Geometry check sheet. Reference: the model listing, model coordinates, mm. Round coordinates to 2 decimals unless told otherwise and drop trailing zeros. Loops run counter-clockwise (first coordinate to the right, second up) from the corner with the lowest first, then second, coordinate; pieces in that order, holes last. Notation, with made-up numbers: (44, -16) -> (64, -16) arc R15 ccw to (64, -8) -> close; hole circle Ø3 at (-32, 88.25). An arc over 180 degrees is marked (long way). Use one line per item in the form item = value.
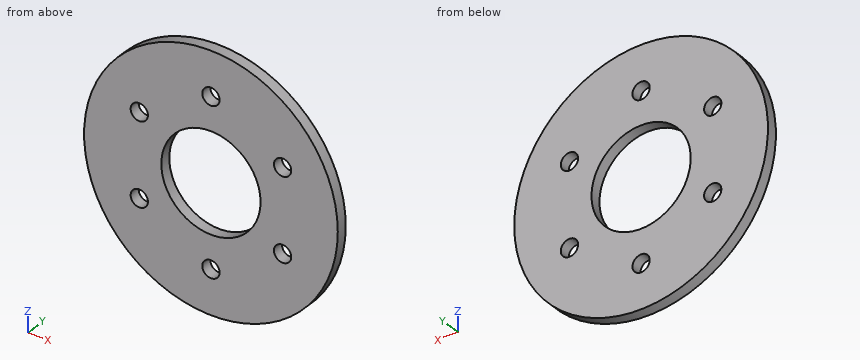
from build123d import *

# Parameters (mm, degrees)
F0_R            = 36.5125
F0_R_2          = 14.2875
F1_DEPTH        = 3.175
F2_R            = 2.4892
F3_DEPTH        = 3.176
F3_COPIES_COUNT = 6


# Not quite as in the source:
# - a pattern or mirror of a feature is missing from the dataset's text; its kind, count and spacing are read off the source's solid


with BuildPart() as f1:
    # F0 (on Front) → F1 (new body)
    with BuildSketch(Plane.XZ):
        Circle(F0_R)
        Circle(F0_R_2, mode=Mode.SUBTRACT)
    extrude(amount=F1_DEPTH)

    # F2 (on face) → F3 (cut, through all)
    with BuildSketch(Plane.XZ.offset(3.175)):
        with Locations((0, 23.8125)):
            Circle(F2_R)
    f3 = extrude(amount=-F3_DEPTH, mode=Mode.SUBTRACT)

    # F3_copies: F3 ×6 about axis
    f3_copies_axis = Axis((0, 0, 0), (0, 1, 0))
    for i in range(1, F3_COPIES_COUNT):
        add(f3.rotate(f3_copies_axis, i * 360 / F3_COPIES_COUNT), mode=Mode.SUBTRACT)


solid = f1.part
1. Section check A-A (x = 0). Record the boundary of the cut face in (y, z) (1 decimal), then the cut area to 3 significant figures.
Return value:
outline = (-3.2, -36.5) -> (0, -36.5) -> (0, -26.3) -> (-3.2, -26.3) -> close; (-3.2, -21.3) -> (0, -21.3) -> (0, -14.3) -> (-3.2, -14.3) -> close; (-3.2, 14.3) -> (0, 14.3) -> (0, 21.3) -> (-3.2, 21.3) -> close; (-3.2, 26.3) -> (0, 26.3) -> (0, 36.5) -> (-3.2, 36.5) -> close
area = 110 mm2
2. Gauge pin test, flat ends, axial feed: pin 1 (4 mm diameter, centred on x = 20.62, z = 11.91, fed in from +Y); pin 2 (1 mm diameter, centred on x = 9, y = -2, fed in from -Z). Record the tip position at first contact, or that the pin passes through.
Return value:
pin_1 = through
pin_2 = -35.51
3. Material ranges on line 1 along Z through (x, y) = (0, -1.5); line 2 along X through (y, z) = (-2.95, -10); line 3 along X through (y, z) = (-2.2, -8.5), recorded low to high.
Return value:
line_1 = -36.51 to -26.3, -21.32 to -14.29, 14.29 to 21.32, 26.3 to 36.51
line_2 = -35.12 to -22.22, -19.02 to -10.2, 10.2 to 19.02, 22.22 to 35.12
line_3 = -35.51 to -11.48, 11.48 to 35.51
4. Section check C-C (y = -1.8). Record the boundary of the cut face in (x, z) (1 decimal).
Return value:
outline = circle Ø73 at (0, 0); hole circle Ø5 at (-20.6, -11.9); hole circle Ø5 at (-20.6, 11.9); hole circle Ø28.6 at (0, 0); hole circle Ø5 at (0, -23.8); hole circle Ø5 at (0, 23.8); hole circle Ø5 at (20.6, -11.9); hole circle Ø5 at (20.6, 11.9)
5. Section check B-B (z = 0). Record the boundary of the cut face in (x, y) (1 decimal), then the cut area to 3 significant figures.
Return value:
outline = (-36.5, -3.2) -> (-14.3, -3.2) -> (-14.3, 0) -> (-36.5, 0) -> close; (14.3, -3.2) -> (36.5, -3.2) -> (36.5, 0) -> (14.3, 0) -> close
area = 141 mm2
6. Section check D-D (x = 10.5). Record the boundary of the cut face in (y, z) (3 decimals), then the cut area to 3 significant figures.
Return value:
outline = (-3.175, -34.97) -> (0, -34.97) -> (0, -9.689) -> (-3.175, -9.689) -> close; (-3.175, 9.689) -> (0, 9.689) -> (0, 34.97) -> (-3.175, 34.97) -> close
area = 161 mm2
